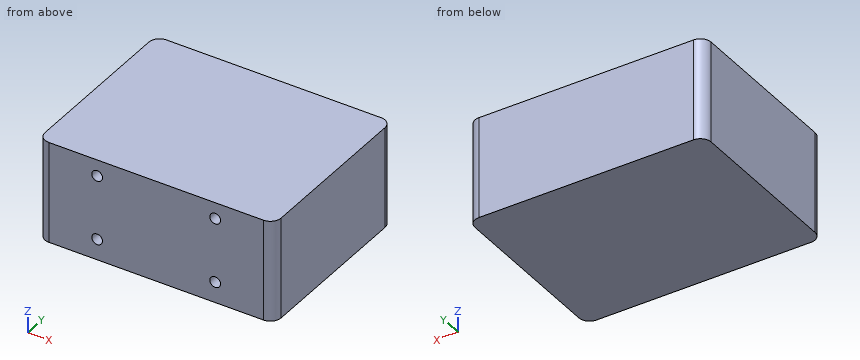
from build123d import *

# Parameters (mm, degrees)
SKETCH1_W           = 44
SKETCH1_H           = 18.9
BOSS_EXTRUDE1_DEPTH = 34
FILLET1_R           = 2
SKETCH2_R           = 1
CUT_EXTRUDE1_DEPTH  = 3.5


with BuildPart() as part:
    # Sketch1 → Boss-Extrude1 (new body)
    with BuildSketch(Plane(origin=(0, 0, 0), x_dir=(1, 0, 0), z_dir=(0, 1, 0))):
        with Locations((22, 9.45)):
            Rectangle(SKETCH1_W, SKETCH1_H)
    extrude(amount=BOSS_EXTRUDE1_DEPTH)

    # Fillet1
    fillet1_edges = [part.edges().sort_by_distance(p)[0] for p in [
        (44, 34, -9.45),
        (0, 34, -9.45),
        (44, 0, -9.45),
        (0, 0, -9.45),
    ]]
    fillet(fillet1_edges, radius=FILLET1_R)

    # Sketch2 → Cut-Extrude1 (cut)
    with BuildSketch(Plane(origin=(0, 0, 0), x_dir=(-1, 0, 0), z_dir=(0, -1, 0))):
        with Locations((-11, 3.02)):
            Circle(SKETCH2_R)
        with Locations((-33, 3.02)):
            Circle(SKETCH2_R)
        with Locations((-11, 15.02)):
            Circle(SKETCH2_R)
        with Locations((-33, 15.02)):
            Circle(SKETCH2_R)
    extrude(amount=-CUT_EXTRUDE1_DEPTH, mode=Mode.SUBTRACT)


solid = part.part
CAD build for the part. Positions are in the model's coordinates, mm. Coordinates: 2 decimals unless noted, no trailing zeros. Loops run counter-clockwise (first coordinate to the right, second up) from the corner with the lowest first, then second, coordinate; pieces in that order, holes last. Notation, with made-up numbers: (83.5, -39) -> (130.5, -39) arc R22 cw to (130.5, 0) -> close; hole circle Ø2 at (-23.5, 48.5). An arc over 180 degrees is marked (long way). One line per item, written item: value.
1. Slice it at B-B on x = 33. Write the cut outline in (y, z), and give its area (3 significant figures).
Answers:
outline: (0, -18.9) -> (34, -18.9) -> (34, 0) -> (0, 0) -> (0, -2.02) -> (3.5, -2.02) -> (3.5, -4.02) -> (0, -4.02) -> (0, -14.02) -> (3.5, -14.02) -> (3.5, -16.02) -> (0, -16.02) -> close
area: 629 mm^2
2. Slice it at A-A on y = 2.5. Write the cut outline in (x, z), and give its area (3 significant figures).
Answers:
outline: (0, -18.9) -> (44, -18.9) -> (44, 0) -> (0, 0) -> close; hole circle Ø2 at (11, -15.02); hole circle Ø2 at (11, -3.02); hole circle Ø2 at (33, -15.02); hole circle Ø2 at (33, -3.02)
area: 819 mm^2
3. Flat gauge pins, fed straight in: P1, Ø2.5, axis at x = 33, z = -3.02, coming from the -Y side; P2, Ø1, axis at x = 33, z = -15, coming from the -Y side. Where does each tip first touch, or does it go through?
Answers:
P1: stops at y = 0
P2: stops at y = 3.5
4. Drill centre lines: line 1 (Z direction, x = 11, y = 1.7); line 2 (X direction, y = 2.3, z = -3.02); line 3 (X direction, y = 1.45, z = -3.02). Where is each one in solid material? Low to high. Write a range as [from, to].
Answers:
line 1: z = [-18.9, -16.02], [-14.02, -4.02], [-2.02, 0]
line 2: x = [0, 10], [12, 32], [34, 44]
line 3: x = [0.08, 10], [12, 32], [34, 43.92]
